Input: part model. Units: mm. Frame: model coordinates. A direction names the side the tool comes from. Coordinates: 2 decimals unless noted, no trailing zeros. Loops run counter-clockwise (first coordinate to the right, second up) from the corner with the lowest first, then second, coordinate; pieces in that order, holes last. Notation, with made-up numbers: (-32.75, 31.5) - (7.25, 31.5) arc R17 cw to (7.25, 47.5) - close; hole circle Ø3 at (-32, 83.25). An arc over 180 degrees is marked (long way). Use a Markdown table: item, result. Add a question column.
1. Ray query, L1, parallel to Y at x = 2.7, z = -4; L2, parallel to X at y = 12, z = -1; L3, parallel to Y at x = 1.4, z = -25.5. Return the intervals inside material, ascending. Write a range as [from, to].
2. Contact query for a flat-ended pin moving along its axis: P1, Ø1.6, axis at x = -4, y = 13, coming from the -Z side. Output: stop coordinate, or through.
3. Draft query along Y for faces 1 (the face through (-3, 13, 1.979)), 2 (the face through (-7.328, 5.956, -3.405)), 3 (the face through (1, 0, -10)). Return one class per face: released by +Y, released by -Y, zero draft, split by the parting line, or undercut.
4. Section query C-C on z = 2.5. Return the cut outline in (x, y), then the cut area to 3 significant figures.
5. Section query A-A on y = 16. Return the cut outline in (x, z).
6. Access query for faces 4 (the face through (-2, 15, 6.979)), 5 (the face through (0, 15, -7)). Directions: +Z, -Z, +X, -X, +Y, -Y. A direction counts if a zero-diameter tool reaches every point of the face in a straight line with its end or side. Return the directions, or none.
7. Section query B-B on z = -25.5. Return the cut outline in (x, y), then the cut area to 4 significant figures.
8. Section query D-D on x = -7.75. Return the cut outline in (y, z), then the cut area to 3 significant figures.
Autodesk Inventor part; units mm, degrees
ref_plane "Work Plane2" through (-5, 31, -22.5) normal (0, 1, 0) x (0, 0, 1)
ref_plane "YZ Plane" through (0, 0, 0) normal (1, 0, 0) x (0, 1, 0)
ref_plane "XZ Plane" through (0, 0, 0) normal (0, 1, 0) x (-1, 0, 0)
ref_plane "Work Plane1" through (0, 0, -31.5) normal (0, -1, 0) x (1, 0, 0)
sketch "Sketch1" plane through (0, 0, -31.5) normal (0, -1, 0) x (1, 0, 0)
  line L0 (0, 31.5) -> (0, 0)
  line L1 (5, 26.9723) -> (5, 36.5)
  line L2 (-5, 0) -> (-5, 31.5)
  line L3 (0, 31.5) -> (-5, 31.5)
  line L4 (5, 3.4786) -> (0, 3.4786)
  line L5 (0, 3.4786) -> (0, 38.4786)
  line L6 (0, 38.4786) -> (5, 38.4786)
  line L7 (5, 38.4786) -> (5, 3.4786)
  line L8 (0, 38.4786) -> (-9.3, 38.4786)
  line L9 (-9.3, 38.4786) -> (-9.3, 33.4786)
  line L10 (-9.3, 33.4786) -> (0, 33.4786)
  line L11 (0, 33.4786) -> (0, 38.4786)
  line L12 (-5.3, 3.4786) -> (-9.3, 3.4786)
  line L13 (-9.3, 3.4786) -> (-9.3, 33.4786)
  line L14 (-9.3, 33.4786) -> (-5.3, 33.4786)
  line L15 (-5.3, 33.4786) -> (-5.3, 3.4786)
  dimension "d0" = 35
  dimension "d1" = 5
  dimension "d2" = 4
  dimension "d3" = 0
  dimension "d4" = 0.3
  dimension "d5" = 0
ref_plane "Work Plane2" through (-5, 31, -22.5) normal (0, 1, 0) x (0, 0, 1)
extrude "Extrusion1" add sketch "Sketch1" against normal up to surface (31 mm away)
sketch "Sketch2" plane through (-9.3, 0, -28.0214) normal (-1, 0, 0) x (0, 0, 1)
  arc A0 (11.8709, 3.8471) -> (24.1214, 10.9199) centre (13.0214, 16) ccw
  line L0 (11.8709, 3.8471) -> (3.0166, 8.9591)
  arc A1 (3.0166, 23.0409) -> (3.0166, 8.9591) centre (13.0214, 16) ccw
  line L1 (3.0166, 23.0409) -> (11.5786, 27.9842)
  arc A2 (24.1214, 20.7426) -> (11.5786, 27.9842) centre (13.0214, 16) ccw
  line L2 (24.1214, 20.7426) -> (24.1214, 10.9199)
  line L3 (-3.4786, 32) -> (-3.4786, -6)
  line L4 (-3.4786, -6) -> (28.0214, -6)
  line L5 (28.0214, -6) -> (28.0214, 32)
  line L6 (-3.4786, 32) -> (28.0214, 32)
  circle A3 centre (13.0214, 16) radius 7.5
  point P0 (28.0214, 0)
  dimension "d8" = 15
extrude "Extrusion2" cut sketch "Sketch2" against normal through all contours A3
sketch "Sketch3" plane through (5, 0, 6.9786) normal (1, 0, 0) x (0, 0, -1)
  arc A0 (6.1231, 27.7) -> (5.1231, 28.7) centre (5.1231, 27.7) ccw
  line L0 (5.1231, 28.7) -> (1.9786, 28.7)
  line L1 (1.9786, 28.7) -> (1.9786, 3)
  line L2 (1.9786, 3) -> (11.5063, 3)
  arc A1 (11.5063, 3) -> (12.5063, 4) centre (11.5063, 4) ccw
  line L3 (12.5063, 4) -> (12.5063, 5.8624)
  arc A2 (13.5063, 6.8624) -> (12.5063, 5.8624) centre (13.5063, 5.8624) ccw
  line L4 (13.5063, 6.8624) -> (31.9786, 6.8624)
  line L5 (31.9786, 6.8624) -> (31.9786, 18.397)
  arc A3 (32.9786, 19.397) -> (31.9786, 18.397) centre (32.9786, 18.397) ccw
  line L6 (32.9786, 19.397) -> (33.9786, 19.397)
  arc A4 (33.9786, 19.397) -> (34.9786, 20.397) centre (33.9786, 20.397) ccw
  line L7 (34.9786, 20.397) -> (34.9786, 22.9624)
  arc A5 (34.9786, 22.9624) -> (33.9786, 23.9624) centre (33.9786, 22.9624) ccw
  line L8 (33.9786, 23.9624) -> (7.1231, 23.9624)
  arc A6 (6.1231, 24.9624) -> (7.1231, 23.9624) centre (7.1231, 24.9624) ccw
  line L9 (6.1231, 24.9624) -> (6.1231, 27.7)
  line L10 (14.4786, 22) -> (29.9786, 22)
  line L11 (29.9786, 22) -> (29.9786, 8.5)
  line L12 (29.9786, 8.5) -> (14.4786, 8.5)
  line L13 (14.4786, 8.5) -> (14.4786, 22)
  circle A7 centre (4.4786, 26) radius 1
  circle A8 centre (10.9786, 5.5) radius 1
  circle A9 centre (32.4786, 21) radius 1
  point P0 (6.9786, 0)
hole "Hole1" at (5, 5.5, -4) at (5, 26, 2.5) at (5, 21, -25.5) direction (-1, 0, 0) diameter 1.5 end through all
sketch "Sketch4" plane through (-9.3, 0, -28.0214) normal (-1, 0, 0) x (0, 0, 1)
  circle A0 centre (30.5214, 26) radius 0.75
  circle A1 centre (24.0214, 5.5) radius 0.75
  circle A2 centre (2.5214, 21) radius 0.75
  circle A3 centre (13.0214, 16) radius 7.5
  line L0 (35, 31) -> (0, 31)
  line L1 (0, 0) -> (0, 31)
  line L2 (35, 0) -> (0, 0)
  line L3 (35, 0) -> (35, 31)
  circle A4 centre (4.8624, 3.8221) radius 1.45
  circle A5 centre (4.8624, 27.0062) radius 1.45
  point P0 (28.0214, 0)
  dimension "d18" = 2.9
  dimension "d19" = 2.9
extrude "Extrusion3" cut sketch "Sketch4" against normal through all contours A4 | A5
properties part number "cellSTORM_inverted_spacerblock_KES400"
Resolved:
| question | item | result |
|---|---|---|
| 1 | L1 | [0, 4.75], [6.25, 31] |
| 1 | L2 | [-9.3, -5.3], [0, 5] |
| 1 | L3 | [0, 20.25], [21.75, 31] |
| 2 | P1 | z = 1.98 |
| 3 | face 1 | zero draft |
| 3 | face 2 | undercut |
| 3 | face 3 | released by -Y |
| 4 | outline | (-9.3, 0) - (5, 0) - (5, 25.25) - (-9.3, 25.25) - close; (-9.3, 26.75) - (5, 26.75) - (5, 31) - (-9.3, 31) - close |
| 4 | area | 422 mm² |
| 5 | outline | (-9.3, -28.02) - (-5.3, -28.02) - (-5.3, -22.5) - (-9.3, -22.5) - close; (-9.3, -7.5) - (-5.3, -7.5) - (-5.3, 1.98) - (0, 1.98) - (0, -7.5) - (5, -7.5) - (5, 6.98) - (-9.3, 6.98) - close; (0, -28.02) - (5, -28.02) - (5, -22.5) - (0, -22.5) - close |
| 6 | face 4 | +Z, +X, -X, +Y, -Y |
| 6 | face 5 | -Z, +Y, -Y |
| 7 | outline | (-9.3, 0) - (-5.3, 0) - (-5.3, 20.25) - (-9.3, 20.25) - close; (-9.3, 21.75) - (-5.3, 21.75) - (-5.3, 31) - (-9.3, 31) - close; (0, 0) - (5, 0) - (5, 20.25) - (0, 20.25) - close; (0, 21.75) - (5, 21.75) - (5, 31) - (0, 31) - close |
| 7 | area | 265.5 mm² |
| 8 | outline | (0, -28.02) - (31, -28.02) - (31, 6.98) - (0, 6.98) - close; hole circle Ø2.9 at (3.82, -23.16); hole circle Ø1.5 at (5.5, -4); hole circle Ø15 at (16, -15); hole circle Ø1.5 at (21, -25.5); hole circle Ø1.5 at (26, 2.5); hole circle Ø2.9 at (27.01, -23.16) |
| 8 | area | 890 mm² |
